Work out the finished part from the listing and answer in its coordinate system (mm). A direction names the side the tool comes from. Coordinates: 2 decimals unless noted, no trailing zeros. Loops run counter-clockwise (first coordinate to the right, second up) from the corner with the lowest first, then second, coordinate; pieces in that order, holes last. Notation, with made-up numbers: (85, 88) - (108, 88) arc R19 ccw to (108, 99) - close; hole circle Ø2 at (6, -34). An arc over 180 degrees is marked (long way). Write each question's results on one line, items separated by ' | '. Start each with the question number.
1. Which of the six approach directions +Z, -Z, +X, -X, +Y, -Y give full straight-line access (tool end or side, diameter ignored) to faces 1 (the cylindrical face through (6.094, 35.325, -0.268)), 2 (the cylindrical face through (-15.24, 32.51, -6.32)), 3 (the cylindrical face through (-8.778, 26.042, -4.524))?
2. A cutting plane is placed at B-B on y = 10.5. Determine the outline of the cut face in (x, z), then the cut area to 3 significant figures.
3. Each of these flat-tipped pins is pushed along its axis until it touches: P1, Ø1.5, axis at y = 27, z = -9, coming from the -X side; P2, Ø3, axis at x = 14, y = 20.5, coming from the +Z side; P3, Ø4, axis at x = -16, y = 16.5, coming from the +Z side; P4, Ø10, axis at x = -0.5, z = 0.5, coming from the +Y side. Where does it stop, or does it pass through?
4. Find the intervals of material crossed by line 1 along Z through (x, y) = (0, 30.5); line 2 along Y through (x, z) = (11.5, -2.5); line 3 along X through (y, z) = (41.5, -5) (3 decimals), in increasing order. Write a range as [from, to].
5. Determine the mould class of faces 4 (the flat face through (-9.9, 33, -18.2)), 5 (the cylindrical face through (1.73, 48.21, -7.81)), 6 (the cylindrical face through (-0.369, 26.042, 9.827)) for opening direction Z: released by +Z, released by -Z, zero draft, split by the parting line, or undercut.
Autodesk Inventor part; units mm, degrees
ref_plane "YZ Plane" through (0, 0, 0) normal (1, 0, 0) x (0, 1, 0)
ref_plane "XZ Plane" through (0, 0, 0) normal (0, 1, 0) x (-1, 0, 0)
ref_plane "XY Plane" through (0, 0, 0) normal (0, 0, 1) x (1, 0, 0)
sketch "Sketch1" plane through (0, 0, 0) normal (0, 0, 1) x (1, 0, 0)
  line L0 (-6.4, 63) -> (-6.4, 48)
  line L1 (-6.4, 48) -> (-6.1, 48)
  line L2 (-6.1, 48) -> (-6.1, 23)
  line L3 (-6.1, 23) -> (-17.5, 23)
  line L4 (-17.5, 23) -> (-17.5, 0)
  line L5 (-17.5, 0) -> (-18.4445, 0)
  line L6 (-18.4445, 0) -> (-22.5, 23)
  line L7 (-22.5, 23) -> (-22.5, 33)
  line L8 (-22.5, 33) -> (-20.5, 33)
  line L9 (-20.5, 33) -> (-20.5, 32)
  line L10 (-20.5, 32) -> (-16.5, 32)
  line L11 (-16.5, 32) -> (-16.5, 33)
  line L12 (-16.5, 33) -> (-8, 33)
  line L13 (-8, 33) -> (-8, 63)
  line L14 (-8, 63) -> (-6.4, 63)
  line L15 (0, -12.6) -> (0, 75.6)
  point P0 (0, 0)
  point P1 (-17.9722, 0)
  dimension "d0" = 23
  dimension "d1" = 15
  dimension "d2" = 30
  dimension "d3" = 10
  dimension "d4" = 17.5
  dimension "d5" = 6.1
  dimension "d6" = 6.4
  dimension "d7" = 8
  dimension "d8" = 22.5
  dimension "d9" = 10
  dimension "d10" = 4
  dimension "d11" = 20.5
  dimension "d12" = 1
revolve "Revolution1" add sketch "Sketch1" angle 360 about axis through (0, -10, 0) along (0, 1, 0)
sketch "Sketch2" plane through (0, 23, 0) normal (0, -1, 0) x (1, 0, 0)
  circle A0 centre (0, 0) radius 11 construction
  point P0 (0, 11)
  point P1 (-9.5263, -5.5)
  point P2 (9.5263, -5.5)
  dimension "d14" = 22
  dimension "d15" = 120
  dimension "d16" = 120
hole "Hole1" at (0, 23, 11) at (-9.5263, 23, -5.5) at (9.5263, 23, -5.5) direction (0, 1, 0) diameter 2.459 depth 6 tip angle 118
properties part number "FlangeCone" material "Brass"
Values:
1) face 1: +Y, -Y | face 2: +Y | face 3: -Y
2) outline: circle Ø40.59 at (0, 0); hole circle Ø35 at (0, 0) | area: 332 mm^2
3) P1: x = -20.93 | P2: z = 18.22 | P3: z = 16.19 | P4: through
4) line 1: [-22.5, -6.1], [6.1, 22.5] | line 2: [23, 33] | line 3: [-6.245, -3.494], [3.494, 6.245]
5) face 4: zero draft | face 5: split by the parting line | face 6: undercut
